```python
from build123d import *

# Parameters (mm, degrees)
EXTRUDE_1_DEPTH            = 460
SKETCH_2_W                 = 6
SKETCH_2_H                 = 10
PATTERN_LINEAR_1_COUNT     = 2
PATTERN_LINEAR_1_PITCH     = 405
PATTERN_LINEAR_1_COL_COUNT = 2
PATTERN_LINEAR_1_COL_PITCH = 405


with BuildPart() as part:
    # 草图1 → 凸台-拉伸1 (new, symmetric)
    with BuildSketch(Plane.XY):
        with BuildLine():
            Line((0, 140), (0, 15))
            ThreePointArc((0, 15), (4.393398282, 4.393398282), (15, 0))
            Line((15, 0), (80, 0))
            Line((80, 0), (80, 10))
            Line((80, 10), (15, 10))
            ThreePointArc((15, 10), (11.464466094, 11.464466094), (10, 15))
            Line((10, 15), (10, 140))
            Line((10, 140), (0, 140))
        make_face()
    extrude(amount=EXTRUDE_1_DEPTH, both=True)

    # 草图2 → 切除-旋转1 (revolve, cut)
    with BuildSketch(Plane.XY, mode=Mode.PRIVATE) as cut_revolve_1_sk:
        with Locations((41, 5)):
            Rectangle(SKETCH_2_W, SKETCH_2_H)
    cut_revolve_1 = revolve(cut_revolve_1_sk.sketch.rotate(Axis((38, 38.728286981, 0), (0, -1, 0)), 180), axis=Axis((38, 38.728286981, 0), (0, -1, 0)), mode=Mode.SUBTRACT)

    # 阵列(线性)1: 切除-旋转1 ×2
    with Locations(*[(0, 0, i * PATTERN_LINEAR_1_PITCH) for i in range(1, PATTERN_LINEAR_1_COUNT)]):
        add(cut_revolve_1, mode=Mode.SUBTRACT)

    # 阵列(线性)1 col: 切除-旋转1 ×2
    with Locations(*[(0, 0, -i * PATTERN_LINEAR_1_COL_PITCH) for i in range(1, PATTERN_LINEAR_1_COL_COUNT)]):
        add(cut_revolve_1, mode=Mode.SUBTRACT)


solid = part.part
```
Input: part model. Units: mm. Frame: model coordinates. A direction names the side the tool comes from. Give positions to 0.01 mm unless a question says otherwise; leave off trailing zeros. Order: outer loops, then holes, each group sorted by start corner. A loop starts at its lowest first (then second) coordinate and runs counter-clockwise, first axis right, second up.
1. Section B-B on y = 50. Return the cut outline in (x, z), and give its area (3 significant figures).
Derived:
outline: (0, -460) - (10, -460) - (10, 460) - (0, 460) - close
area: 9,200 mm2
2. Reachability of faces 1 (the flat face through (48, 10, 6)), 2 (the flat face through (7, 50, 460)) from +Z, -Z, +X, -X, +Y, -Y: full face, straight path, thin tool, end or side. Return the list, or none.
Derived:
face 1: +Z, -Z, +X, +Y
face 2: +Z, +X, -X, +Y, -Y
3. Material intervals for L1, parallel to Z at x = 38, y = 3.75; L2, parallel to Y at x = 44, z = 86, sorted ascending.
Derived:
L1: z = -460 to -411, -399 to -6, 6 to 399, 411 to 460
L2: y = 0 to 10
4. Section A-A on z = 268.5. Return the cut outline in (x, y).
Derived:
outline: (0, 15) arc R15 ccw to (15, 0) - (80, 0) - (80, 10) - (15, 10) arc R5 cw to (10, 15) - (10, 140) - (0, 140) - close
5. Pin query (flat end, axial travel): pin 1 (15.5 mm diameter, centred on x = 38, z = -405, fed in from +Y); pin 2 (3 mm diameter, centred on y = 14, z = -30.5, fed in from +X); pin 3 (14 mm diameter, centred on x = 38, z = 405, fed in from -Y); pin 4 (4 mm diameter, centred on x = 8.5, z = 254, fed in from -Y). Return the tip coordinate at first contact, or that it passes through.
Derived:
pin 1: stops at y = 10
pin 2: stops at x = 10.67
pin 3: stops at y = 0
pin 4: stops at y = 0.69
